Design review of the part built by this model. Coordinates are the model's own, in mm. A direction names the side the tool comes from. Give positions to 0.01 mm unless a question says otherwise; leave off trailing zeros. Loops run counter-clockwise (first coordinate to the right, second up) from the corner with the lowest first, then second, coordinate; pieces in that order, holes last. Notation, with made-up numbers: (40, 36.25) -> (75, 36.25) arc R22 cw to (75, 59.25) -> close; hole circle Ø4 at (48.5, 8.5). An arc over 180 degrees is marked (long way). Answer as CSV lines item,"result".
Autodesk Inventor part; units mm, degrees
ref_plane "YZ Plane" through (0, 0, 0) normal (1, 0, 0) x (0, 1, 0)
ref_plane "XZ Plane" through (0, 0, 0) normal (0, 1, 0) x (-1, 0, 0)
ref_plane "XY Plane" through (0, 0, 0) normal (0, 0, 1) x (1, 0, 0)
sketch "Sketch1" plane through (0, 0, 0) normal (0, 1, 0) x (-1, 0, 0)
  line L0 (1.6318, 52.1856) -> (-109.4932, 52.1856)
  line L1 (-109.4932, 52.1856) -> (-109.4932, -4.9644)
  line L2 (-109.4932, -4.9644) -> (1.6318, -4.9644)
  line L3 (1.6318, -4.9644) -> (1.6318, 52.1856)
  point P0 (0, 0)
extrude "Extrusion1" add sketch "Sketch1" along normal blind 39.6875
sketch "Sketch2" plane through (0, 39.6875, 0) normal (0, 1, 0) x (1, 0, 0)
  line L0 (-0.0443, -50.5981) -> (107.9057, -50.5981)
  line L1 (107.9057, -50.5981) -> (107.9057, 3.3769)
  line L2 (107.9057, 3.3769) -> (-0.0443, 3.3769)
  line L3 (-0.0443, 3.3769) -> (-0.0443, -50.5981)
  line L4 (-1.6318, -52.1856) -> (109.4932, -52.1856)
  line L5 (109.4932, 4.9644) -> (-1.6318, 4.9644)
  line L6 (-1.6318, 4.9644) -> (-1.6318, -52.1856)
  line L7 (109.4932, -52.1856) -> (109.4932, 4.9644)
  point P0 (0, 0)
  dimension "d8" = 1.5875
  dimension "d9" = 1.5875
  dimension "d10" = 1.5875
  dimension "d11" = 1.5875
extrude "Extrusion2" cut sketch "Sketch2" against normal blind 36.5125 contours L3 L2 L1 L0
sketch "Sketch3" plane through (109.4932, 0, 52.1856) normal (1, 0, 0) x (0, 0, -1)
  line L0 (10.3187, 19.05) -> (23.0187, 19.05)
  line L1 (23.0187, 19.05) -> (23.0187, 7.9375)
  line L2 (23.0187, 7.9375) -> (10.3187, 7.9375)
  line L3 (10.3187, 7.9375) -> (10.3187, 19.05)
  line L4 (0, 0) -> (57.15, 0)
  line L5 (0, 0) -> (0, 39.6875)
  line L6 (7.9375, 38.1) -> (24.6062, 38.1)
  line L7 (24.6062, 38.1) -> (24.6062, 23.8125)
  line L8 (24.6062, 23.8125) -> (7.9375, 23.8125)
  line L9 (7.9375, 23.8125) -> (7.9375, 38.1)
  line L10 (0, 39.6875) -> (57.15, 39.6875)
  line L11 (55.5625, 3.175) -> (1.5875, 3.175)
  line L12 (1.5875, 39.6875) -> (1.5875, 3.175)
  point P0 (52.1856, 0)
  point P1 (55.5625, 39.6875)
  point P2 (1.5875, 0)
  dimension "d14" = 12.7
  dimension "d15" = 11.1125
  dimension "d18" = 16.6687
  dimension "d19" = 14.2875
  dimension "d23" = 4.7625
  dimension "d28" = 4.7625
  dimension "d29" = 8.7312
  dimension "d30" = 6.35
  dimension "d34" = 1.5875
extrude "Extrusion3" cut sketch "Sketch3" against normal up to surface (1.5875 mm away)
properties part number "SD_BaseStation_Box"
Q1. We need section B-B, the plane y = 20.5. State the section outline as (x, z) points.
Filled sheet:
outline,"(-1.63, -4.96) -> (109.49, -4.96) -> (109.49, 52.19) -> (-1.63, 52.19) -> close; hole (-0.04, -3.38) -> (107.91, -3.38) -> (107.91, 50.6) -> (-0.04, 50.6) -> close"
Q2. To check wall thickness, follow probe 1 along Z at (x, y) = (52.5, 23); probe 2 along X at (y, z) = (29.5, 46.5); probe 3 along Y at (x, z) = (9, 13.5) (3 decimals). State the ranges of each line that lie inside material, in increasing order. Write a range as from..to.
Filled sheet:
probe 1,"z = -4.96..-3.38, 50.6..52.19"
probe 2,"x = -1.63..-0.04, 107.91..109.49"
probe 3,"y = 0..3.175"
Q3. Clearance check with flat-ended pins moving along their axes: pin 1 Ø1 at (y, z) = (34.5, 33) entering from +X; pin 2 Ø16 at (x, z) = (59.5, 20) entering from +Y (3 decimals). State where each tip first meets the part, or that it passes through.
Filled sheet:
pin 1,"stops at x = -0.04"
pin 2,"stops at y = 3.175"
Q4. We need section A-A, the plane z = 39. State how many separate pieces and enclosed holes the cut face has, and give its area (3 significant figures).
Filled sheet:
separate pieces,"3"
enclosed holes,"0"
area,"428 mm^2"
Q5. The part is to be moulded in two halves that separate along X. For faces 3 (the flat face through (53, 3.175, 23)), 4 (the flat face through (53, 20, 52.186)), 5 (the flat face through (-1.632, 20, 23)), say which applies: pulls with the +X half, pulls with the -X half, needs draft (parallel to the pull), parting line crosses it, or undercut.
Filled sheet:
face 3,"undercut"
face 4,"needs draft"
face 5,"pulls with the -X half"
Q6. We need section D-D, the plane x = 39. State the section outline as (y, z) points (1 decimal).
Filled sheet:
outline,"(0, -5) -> (39.7, -5) -> (39.7, -3.4) -> (3.2, -3.4) -> (3.2, 50.6) -> (39.7, 50.6) -> (39.7, 52.2) -> (0, 52.2) -> close"
Q7. We need section C-C, the plane z = 26. State the section outline as (x, y) points (1 decimal).
Filled sheet:
outline,"(-1.6, 0) -> (109.5, 0) -> (109.5, 39.7) -> (107.9, 39.7) -> (107.9, 3.2) -> (0, 3.2) -> (0, 39.7) -> (-1.6, 39.7) -> close"
Q8. For faces 1 (the flat face through (-0.044, 22, 23)), 2 (the flat face through (54, 39.688, 51)), list the 3-axis set-ups (+Z, -Z, +X, -X, +Y, -Y) from which the entire face can be reached by the end or side of a thin tool; tool diameter is ignored.
Filled sheet:
face 1,"+Y"
face 2,"+Z, -Z, +X, -X, +Y"
